```python
from build123d import *

# Parameters (mm, degrees)
BOSS_EXTRUDE1_DEPTH = 2.38
BOSS_EXTRUDE2_DEPTH = 10
BOSS_EXTRUDE3_DEPTH = 2.38
BOSS_EXTRUDE4_DEPTH = 2.38
SKETCH5_R           = 2.75
CUT_EXTRUDE1_DEPTH  = 178.5
SKETCH6_R           = 2.75
CUT_EXTRUDE2_DEPTH  = 20.88


with BuildPart() as part:
    # Sketch1 → Boss-Extrude1 (new body)
    with BuildSketch(Plane.XY):
        with BuildLine():
            Line((0, 0), (177.5, 0))
            Line((177.5, 0), (177.5, 138.75))
            ThreePointArc((177.5, 138.75), (88.75, 227.5), (0, 138.75))
            Line((0, 138.75), (0, 0))
        make_face()
    extrude(amount=BOSS_EXTRUDE1_DEPTH)

    # Sketch2 → Boss-Extrude2 (add)
    with BuildSketch(Plane.XY.offset(2.38)):
        with BuildLine():
            Line((175.12, 2.38), (175.12, 138.75))
            ThreePointArc((175.12, 138.75), (88.75, 225.12), (2.38, 138.75))
            Line((2.38, 138.75), (2.38, 2.38))
            Line((2.38, 2.38), (2.38, 0))
            Line((2.38, 0), (0, 0))
            Line((0, 0), (0, 138.75))
            ThreePointArc((0, 138.75), (88.75, 227.5), (177.5, 138.75))
            Line((177.5, 138.75), (177.5, 0))
            Line((177.5, 0), (175.12, 0))
            Line((175.12, 0), (175.12, 2.38))
        make_face()
    extrude(amount=BOSS_EXTRUDE2_DEPTH)

    # Sketch3 → Boss-Extrude3 (add)
    with BuildSketch(Plane(origin=(177.5, 0, 0), x_dir=(0, 0, -1), z_dir=(1, 0, 0))):
        with BuildLine():
            Line((-12.38, 15), (-12.38, 0))
            ThreePointArc((-12.38, 0), (-19.88, 7.5), (-12.38, 15))
        make_face()
    extrude(amount=-BOSS_EXTRUDE3_DEPTH)

    # Sketch4 → Boss-Extrude4 (add)
    with BuildSketch(Plane.ZY):
        with BuildLine():
            Line((12.38, 15), (12.38, 0))
            ThreePointArc((12.38, 0), (19.88, 7.5), (12.38, 15))
        make_face()
    extrude(amount=-BOSS_EXTRUDE4_DEPTH)

    # Sketch5 → Cut-Extrude1 (cut, through all)
    with BuildSketch(Plane.ZY):
        with Locations((12.807918023, 7.485123177)):
            Circle(SKETCH5_R)
    extrude(amount=-CUT_EXTRUDE1_DEPTH, mode=Mode.SUBTRACT)

    # Sketch6 → Cut-Extrude2 (cut, through all)
    with BuildSketch(Plane(origin=(0, 0, 0), x_dir=(-1, 0, 0), z_dir=(0, 0, -1))):
        with Locations((-88.75, 182.5)):
            Circle(SKETCH6_R)
        with Locations((-88.75, 152.5)):
            Circle(SKETCH6_R)
    extrude(amount=-CUT_EXTRUDE2_DEPTH, mode=Mode.SUBTRACT)


solid = part.part
```
For this review, take the finished solid that the model builds, in its own axes (mm). A direction names the side the tool comes from. Coordinates: 2 decimals unless noted, no trailing zeros. Loops run counter-clockwise (first coordinate to the right, second up) from the corner with the lowest first, then second, coordinate; pieces in that order, holes last.
1. Add section D-D, the plane y = 182.5. Give the boundary of the cut face in (x, z), then the cut area to 3 significant figures.
2. For line 1 (Y direction, x = 88.75, z = 0.95); line 2 (X direction, y = 13, z = 6); line 3 (Z direction, x = 129.5, y = 64), list the stretches that pass through material, from the lowest coordinate up.
3. Insertion check: P1, Ø5, axis at y = 7.49, z = 12.81, coming from the -X side; P2, Ø6, axis at x = 34.5, z = 7, coming from the -Y side; P3, Ø2, axis at x = 48, z = 7.5, coming from the +Y side; P4, Ø10, axis at x = 137.5, z = 9, coming from the +Y side. Each pin has a flat end and moves straight along its axis. Give the tip position at first contact, or say it passes through.
4. Mouldability with a two-part tool opening along X and no side actions: class faces 3 (the flat face through (88, 114, 2.38)), 4 (the cylindrical face through (86.8, 227.48, 6.1)), 5 (the flat face through (0, 70, 8)), 6 (the flat face through (109, 224, 12.38)) as +X half, -X half, draft (parallel to the pull), parting line (faces both ways), or undercut.
5. Add section A-A, the plane x = 88.75. Give the boundary of the cut face in (y, z).
6. Add section B-B, the plane z = 5.25. Give the boundary of the cut face in (x, y).
7. For faces 1 (the cylindrical face through (90.932, 180.827, 1.173)), 2 (the cylindrical face through (90.6, 225.1, 7.3)), list the 3-axis set-ups (+Z, -Z, +X, -X, +Y, -Y) from which the entire face can be reached by the end or side of a thin tool; tool diameter is ignored.
8. Add section C-C, the plane y = 128.5. Give the boundary of the cut face in (x, z).
Result:
1. outline: (11.53, 0) - (86, 0) - (86, 2.38) - (14.28, 2.38) - (14.28, 12.38) - (11.53, 12.38) - close; (91.5, 0) - (165.97, 0) - (165.97, 12.38) - (163.22, 12.38) - (163.22, 2.38) - (91.5, 2.38) - close
1. area: 409 mm2
2. line 1: y = 0 to 149.75, 155.25 to 179.75, 185.25 to 227.5
2. line 2: x = 0 to 2.38, 175.12 to 177.5
2. line 3: z = 0 to 2.38
3. P1: passes through
3. P2: stops at y = 203.42
3. P3: stops at y = 218.1
3. P4: stops at y = 215.97
4. face 3: undercut
4. face 4: parting line
4. face 5: -X half
4. face 6: draft
5. outline: (0, 0) - (149.75, 0) - (149.75, 2.38) - (0, 2.38) - close; (155.25, 0) - (179.75, 0) - (179.75, 2.38) - (155.25, 2.38) - close; (185.25, 0) - (227.5, 0) - (227.5, 12.38) - (225.12, 12.38) - (225.12, 2.38) - (185.25, 2.38) - close
6. outline: (0, 0) - (2.38, 0) - (2.38, 138.75) arc R86.37 cw to (175.12, 138.75) - (175.12, 0) - (177.5, 0) - (177.5, 138.75) arc R88.75 ccw to (0, 138.75) - close
7. face 1: +Z, -Z
7. face 2: +Z, -Y
8. outline: (0, 0) - (177.5, 0) - (177.5, 12.38) - (175.12, 12.38) - (175.12, 2.38) - (2.38, 2.38) - (2.38, 12.38) - (0, 12.38) - close
